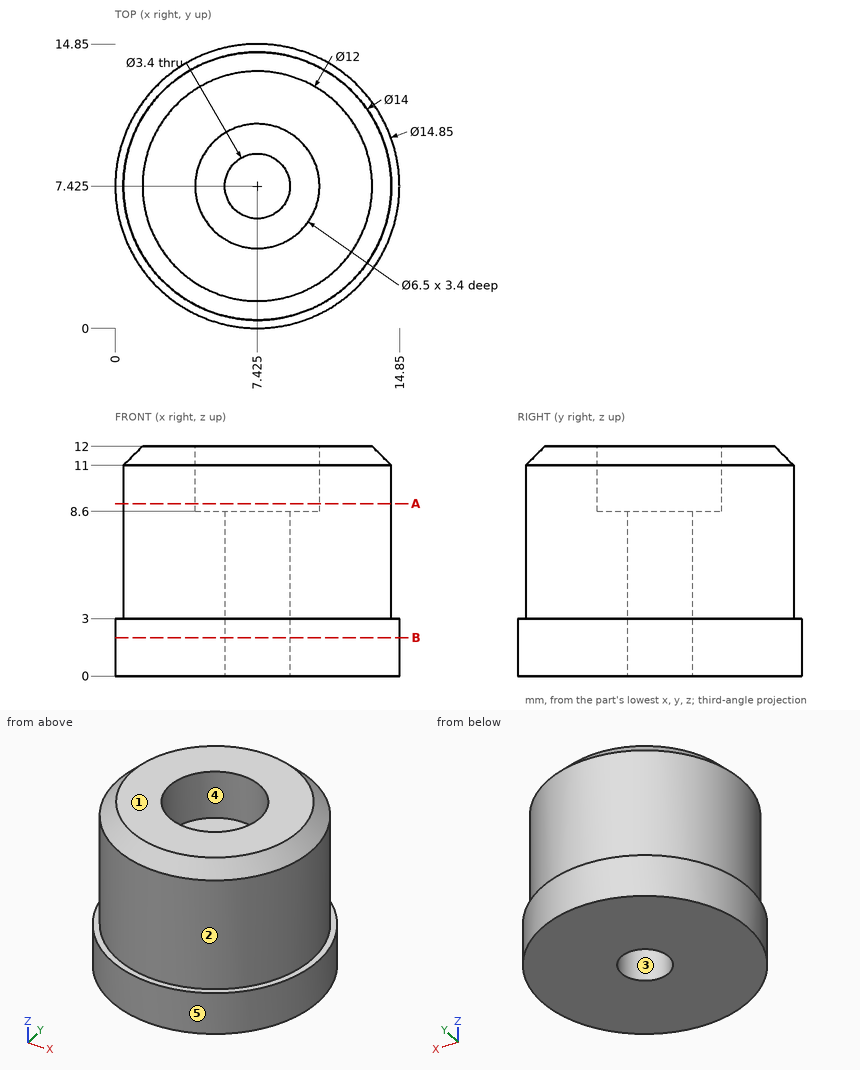
Study the drawing (mm; zero at the part's minimum x, y, z) and answer. A direction names the side the tool comes from. Give positions to 0.01 mm unless a question says otherwise; leave off trailing zeros. Write each loop counter-clockwise with the first axis right and the second up, starting at its lowest first coordinate (ties: lowest second). Pieces come first, ordered by that corner, then holes. Notation, with made-up numbers: M 18,-39.5 L 36,-39.5 A25 ccw 36,-3.5 Z; hole C 84,63.25 d4. An arc over 180 degrees is marked long. Put each result on its own line as item: value. Start each with the question number.
1. The part is cut by section B-B, the plane z = 2. Give the vertices of the cut face in (x, y) (3 decimals).
2. The part is cut by section A-A, the plane z = 9. Give the vertices of the cut face in (x, y) (3 decimals).
3. Each of these flat-tipped pins is pushed along its axis until it touches: pin 1 Ø1.5 at (y, z) = (9, 10.5) entering from +X; pin 2 Ø5 at (x, z) = (12.5, 10) entering from +Y; pin 3 Ø5 at (x, z) = (5.5, 5) entering from +Y. Where does it stop, or does it pass through?
4. Consider line 1 along X through (y, z) = (7.5, 8); line 2 along Z through (x, y) = (5.25, 8); line 3 along Y through (x, z) = (5.75, 8.75). Determine where each line is inside the solid, lowest interval first.
5. For a pull along Y with two mould halves and no side action, classify the marked faces 1, 2 and 3 as released by +Y, released by -Y, zero draft, split by the parting line, or undercut.
6. Which of the six approach directions +Z, -Z, +X, -X, +Y, -Y give full straight-line access (tool end or side, diameter ignored) to the marked faces 4 and 5?
Final values:
1. outline: C 7.425,7.425 d14.85; hole C 7.425,7.425 d3.4
2. outline: C 7.425,7.425 d14; hole C 7.425,7.425 d6.5
3. pin 1: stops at x = 14.38
3. pin 2: stops at y = 13.93
3. pin 3: stops at y = 14.84
4. line 1: x = 0.43 to 5.73, 9.12 to 14.42
4. line 2: z = 0 to 8.6
4. line 3: y = 0.63 to 4.64, 10.21 to 14.22
5. face 1: zero draft
5. face 2: split by the parting line
5. face 3: undercut
6. face 4: +Z
6. face 5: +Z, -Z
